Input: part model. Units: mm. Frame: model coordinates. Round coordinates to 2 decimals unless told otherwise and drop trailing zeros. Loops run counter-clockwise (first coordinate to the right, second up) from the corner with the lowest first, then second, coordinate; pieces in that order, holes last. Notation, with made-up numbers: M 24.25,-11 L 35.25,-11 A34 cw 35.25,24 Z; hole C 1,-18.5 d1. An arc over 180 degrees is marked long. Put each result on its own line as item: value. Start each with the question number.
1) Section B-B on z = 0.5. Output: boundary loops of the cut face in (x, y).
2) Pin query (flat end, axial travel): pin 1 (1 mm diameter, centred on x = 2.5, y = -40.5, fed in from +Z). Return the tip coordinate at first contact, or that it passes through.
3) Section A-A on y = -38.5. Output: boundary loops of the cut face in (x, z).
4) Line query: probe 1 along Z at (x, y) = (-3.5, -28.5); probe 2 along X at (y, z) = (-48.5, 3); probe 3 along X at (y, z) = (-51, 1.2). Output: solid intervals per line, ascending.
5) Section C-C on x = 3.25. Output: boundary loops of the cut face in (y, z).
from build123d import *

# Parameters (mm, degrees)
F1_DEPTH = 60.75
F2_W     = 29.965812
F2_H     = 12.152278
F3_DEPTH = 80


with BuildPart() as f1:
    # F0 (on Front) → F1 (new body)
    with BuildSketch(Plane.XZ):
        with BuildLine():
            ThreePointArc((4.855605, 2.640416), (4.442922, 4.303856), (2.741867, 4.513024))
            ThreePointArc((2.741867, 4.513024), (1.603415, 5.794144), (0, 5.188834))
            ThreePointArc((0, 5.188834), (-1.603415, 5.794144), (-2.741867, 4.513024))
            ThreePointArc((-2.741867, 4.513024), (-4.442922, 4.303856), (-4.855605, 2.640416))
            ThreePointArc((-4.855605, 2.640416), (-6.264609, 1.664686), (-5.856982, 0))
            ThreePointArc((-5.856982, 0), (-6.651149, -1.518762), (-5.516596, -2.803335))
            ThreePointArc((-5.516596, -2.803335), (-5.513992, -4.5172), (-3.912424, -5.12738))
            ThreePointArc((-3.912424, -5.12738), (-3.113645, -6.643722), (-1.411962, -6.439723))
            ThreePointArc((-1.411962, -6.439723), (0, -7.411166), (1.411962, -6.439723))
            ThreePointArc((1.411962, -6.439723), (3.113645, -6.643722), (3.912424, -5.12738))
            ThreePointArc((3.912424, -5.12738), (5.513992, -4.5172), (5.516596, -2.803335))
            ThreePointArc((5.516596, -2.803335), (6.651149, -1.518762), (5.856982, 0))
            ThreePointArc((5.856982, 0), (6.264609, 1.664686), (4.855605, 2.640416))
        make_face()
    extrude(amount=F1_DEPTH)

    # F2 (on Front) → F3 (cut)
    with BuildSketch(Plane.XZ):
        with Locations((-0.254262, -6.076139)):
            Rectangle(F2_W, F2_H)
    extrude(amount=F3_DEPTH, mode=Mode.SUBTRACT)


solid = f1.part
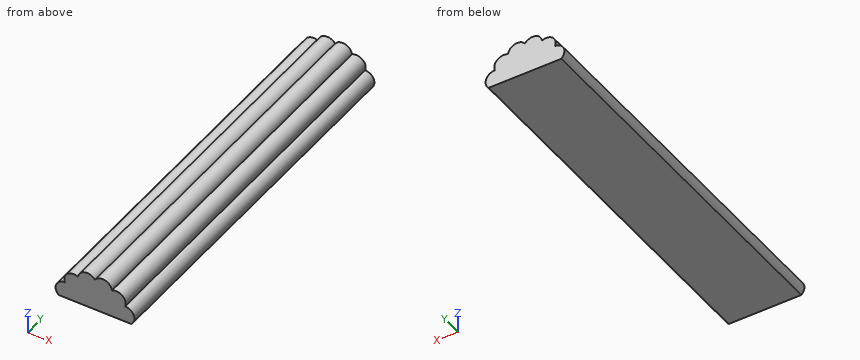
Geometry results:
1. outline: M -6.23,-60.75 L 6.23,-60.75 L 6.23,0 L -6.23,0 Z
2. pin 1: stops at z = 5.63
3. outline: M -5.86,0 L 5.86,0 A1.51 ccw 4.86,2.64 A1.51 ccw 2.74,4.51 A1.51 ccw 0,5.19 A1.51 ccw -2.74,4.51 A1.51 ccw -4.86,2.64 A1.51 ccw Z
4. probe 1: z = 0 to 4.68
4. probe 2: x = -4.94 to 4.94
4. probe 3: x = -6.36 to 6.36
5. outline: M -60.75,0 L 0,0 L 0,4.67 L -60.75,4.67 Z
